The model under review builds one solid part; all positions refer to its coordinate system, in mm. A direction names the side the tool comes from. Coordinates: 2 decimals unless noted, no trailing zeros. Write each loop counter-clockwise with the first axis right and the second up, starting at its lowest first coordinate (ties: lowest second). Pieces come first, ordered by that corner, then holes. Notation, with made-up numbers: (50, 86) - (68, 86) arc R6 ccw to (68, 96) - close; hole circle Ø11 at (-23.75, -30). An arc over 180 degrees is marked (long way). Put each result on its own line as item: value.
from build123d import *

# Parameters (mm, degrees)
SKETCH1_R               = 4.7625
BOSS_EXTRUDE1_DEPTH     = 5.08
SKETCH4_W               = 19.05
SKETCH4_H               = 5.08
BOSS_EXTRUDE2_DEPTH     = 5.08
SKETCH5_R               = 1.660728382
SKETCH5_R_2             = 1.651
CUT_EXTRUDE1_DEPTH      = 1.0000001
CUT_EXTRUDE1_DEPTH_BACK = 6.0800001
SKETCH6_R               = 4.7625
BOSS_EXTRUDE3_DEPTH     = 5.08
CUT_EXTRUDE2_DEPTH      = 1.0000001
CUT_EXTRUDE2_DEPTH_BACK = 6.0800001


with BuildPart() as part:
    # Sketch1 → Boss-Extrude1 (new body)
    with BuildSketch(Plane(origin=(0, 0, 0), x_dir=(1, 0, 0), z_dir=(0, 1, 0))):
        with BuildLine():
            Line((-9.525, 53.975), (9.525, 53.975))
            Line((9.525, 53.975), (9.525, 51.435))
            add(Edge.make_bspline(
                [(9.525, 51.435), (9.525, 51.21454564), (27.819109584, -48.895), (60.325, -48.895)],
                knots=[0, 0, 0, 0, 1, 1, 1, 1], degree=3))
            Line((60.325, -48.895), (-9.525, -48.895))
            Line((-9.525, -48.895), (-9.525, 53.975))
        make_face()
        with Locations((0, 45.9867)):
            Circle(SKETCH1_R, mode=Mode.SUBTRACT)
    extrude(amount=BOSS_EXTRUDE1_DEPTH)

    # Sketch4 → Boss-Extrude2 (add)
    with BuildSketch(Plane(origin=(0, 5.08, 0), x_dir=(1, 0, 0), z_dir=(0, 1, 0))):
        with Locations((50.8, -51.435)):
            Rectangle(SKETCH4_W, SKETCH4_H)
    extrude(amount=-BOSS_EXTRUDE2_DEPTH)

    # Sketch5 → Cut-Extrude1 (cut, two sides)
    with BuildSketch(Plane.XZ) as cut_extrude1_sk:
        with Locations((-0.635, 4.445)):
            Circle(SKETCH5_R)
        with Locations((37.465, 40.005)):
            Circle(SKETCH5_R_2)
    extrude(amount=CUT_EXTRUDE1_DEPTH, mode=Mode.SUBTRACT)
    extrude(cut_extrude1_sk.sketch, amount=-CUT_EXTRUDE1_DEPTH_BACK, mode=Mode.SUBTRACT)

    # Sketch6 → Boss-Extrude3 (add)
    with BuildSketch(Plane.XZ):
        with BuildLine():
            Line((-14.535912, -0.037592), (-9.525, -0.037592))
            Line((-9.525, -0.037592), (-9.525, -1.398441508))
            ThreePointArc((-9.525, -1.398441508), (-4.629912, -9.943592), (-9.525, -18.488742492))
            Line((-9.525, -18.488742492), (-9.525, -19.849592))
            Line((-9.525, -19.849592), (-14.535912, -19.849592))
            ThreePointArc((-14.535912, -19.849592), (-24.441912, -9.943592), (-14.535912, -0.037592))
        make_face()
        with Locations((-14.535912, -9.943592)):
            Circle(SKETCH6_R, mode=Mode.SUBTRACT)
    extrude(amount=-BOSS_EXTRUDE3_DEPTH)

    # Sketch9 → Cut-Extrude2 (cut, two sides)
    with BuildSketch(Plane.XZ) as cut_extrude2_sk:
        with BuildLine():
            Line((60.325, 53.975), (60.325, 48.895))
            add(Edge.make_bspline(
                [(60.325, 48.895), (55.814379896, 48.895), (51.577410685, 46.967369191), (47.625, 43.646486826)],
                knots=[0, 0, 0, 0, 0.138763161, 0.138763161, 0.138763161, 0.138763161], degree=3))
            Line((47.625, 43.646486826), (47.625, 48.895))
            Line((47.625, 48.895), (41.275, 48.895))
            Line((41.275, 48.895), (41.275, 53.975))
            Line((41.275, 53.975), (60.325, 53.975))
        make_face()
    extrude(amount=CUT_EXTRUDE2_DEPTH, mode=Mode.SUBTRACT)
    extrude(cut_extrude2_sk.sketch, amount=-CUT_EXTRUDE2_DEPTH_BACK, mode=Mode.SUBTRACT)


solid = part.part
1. Consider section C-C on y = 2.4. Give the number of separate pieces and of enclosed holes in the cut face, plus the area to 3 significant figures.
Determined:
separate pieces: 1
enclosed holes: 4
area: 3,600 mm^2
2. Machinability: for faces 4 (the flat face through (9.525, 3, -53)), 5 (the flat face through (-12, 3, -19.85)), 6 (the cylindrical face through (39.04, 2.5, 40.5)), 7 (the flat face through (-9.525, 3, 25)), which of the approach directions +Z, -Z, +X, -X, +Y, -Y give a long, thin tool a straight path to every point of the face, cutting with its end or side? Answer none if there is none.
Determined:
face 4: -Z, +X, +Y, -Y
face 5: -Z, -X, +Y, -Y
face 6: +Y, -Y
face 7: +Z, -X, +Y, -Y
3. Consider section B-B on x = 0. State the section outline as (y, z) points (3 decimals), plus the area to 3 significant figures.
Determined:
outline: (0, -53.975) - (5.08, -53.975) - (5.08, -50.749) - (0, -50.749) - close; (0, -41.224) - (5.08, -41.224) - (5.08, 2.91) - (0, 2.91) - close; (0, 5.98) - (5.08, 5.98) - (5.08, 48.895) - (0, 48.895) - close
area: 459 mm^2
4. For pin 1 Ø2.5 at (y, z) = (1.5, -39) entering from -X (3 decimals); pin 2 Ø2 at (y, z) = (4, -9.5) entering from -X; pin 3 Ø3 at (x, y) = (-13.5, 3) entering from -Z; pin 4 Ø2 at (y, z) = (3.5, -52) entering from +X, all flat-tipped, find the tip position at first contact; note any pin that passes through.
Determined:
pin 1: stops at x = -9.525
pin 2: stops at x = -24.44
pin 3: stops at z = -19.85
pin 4: stops at x = 9.6
5. Consider section A-A on x = -11. State the section outline as (y, z) points.
Determined:
outline: (0, -19.85) - (5.08, -19.85) - (5.08, -13.13) - (0, -13.13) - close; (0, -6.75) - (5.08, -6.75) - (5.08, -0.04) - (0, -0.04) - close
6. To check wall thickness, follow probe 1 along Z at (x, y) = (0, 2.05) (3 decimals); probe 2 along Z at (x, y) = (-14, 0.95); probe 3 along Z at (x, y) = (-10.5, 4.05). State the ranges of each line that lie inside material, in increasing order.
Determined:
probe 1: z = -53.975 to -50.749, -41.224 to 2.91, 5.98 to 48.895
probe 2: z = -19.85 to -14.68, -5.21 to -0.04
probe 3: z = -19.85 to -12.47, -7.42 to -0.04
7. The part is to be moulded in two halves that separate along Z. For faces 1 (the flat face through (0, 3, -53.975)), 2 (the flat face through (-9.525, 3, -37)), 3 (the cylindrical face through (-1.032, 2.504, -41.337)), say which applies: +Z half, -Z half, draft (parallel to the pull), parting line (faces both ways), or undercut.
Determined:
face 1: -Z half
face 2: draft
face 3: undercut
